```python
from build123d import *

# Parameters (mm, degrees)
F0_W        = 19.1873764305
F0_H        = 101.6
F1_DEPTH    = 76.2
F3_DEPTH    = 67.31
F4_T1_DEPTH = 697.6501262753
F5_R        = 5.07999
F6_R        = 5.08


# Not quite as in the source:
# - a fillet or chamfer that OpenCascade refuses, or shapes differently, is made with other operations: its cross-section is extruded or revolved along the edge and cut away or added
# - a fillet or chamfer is up to 0.001 mm smaller than in the source, because OpenCascade refuses the exact size


with BuildPart() as f1:
    # F0 (on Right) → F1 (new body, symmetric)
    with BuildSketch(Plane.YZ):
        with BuildLine():
            Line((-28.6442058678, -4.364277937), (-36.9899753063, 5.2085028753))
            Line((-36.9899753063, 5.2085028753), (-36.9899753063, -13.8414971247))
            Line((-36.9899753063, -13.8414971247), (39.2100246937, -13.8414971247))
            Line((39.2100246937, -13.8414971247), (39.2100246937, 87.7585028753))
            ThreePointArc((39.2100246937, 87.7585028753), (20.4155377225, 30.5509785676), (-28.6442058678, -4.364277937))
        make_face()
        Polygon((-36.9899753063, -13.8414971247), (-36.9899753063, 5.2085028753), (-36.9899753063, 5.6934356689), (-42.0699753063, 5.6934356689), (-42.0699753063, -13.8414971247), align=None)
        with Locations((48.803712909, 36.9585028753)):
            Rectangle(F0_W, F0_H)
    extrude(amount=F1_DEPTH, both=True)

    # F2 (on Front) → F3 (cut, symmetric)
    with BuildSketch(Plane.XZ):
        with BuildLine():
            ThreePointArc((50.7993000876, -14.1734545694), (0.1539604747, 36.9344649658), (-50.8002333049, -13.8655350342))
            Line((-50.8002333049, -13.8655350342), (50.7993000876, -14.1734545694))
        make_face()
    extrude(amount=F3_DEPTH, both=True, mode=Mode.SUBTRACT)

    # F4: fillet of radius 319.4825375631 on 1 edges, made by hand

    # F4_s2 → F4_t1 (cut)
    with BuildSketch(Plane.YZ.offset(-348.8250631377)):
        with BuildLine():
            ThreePointArc((39.2100246937, 87.7585028753), (53.5639950587, 34.0710629609), (58.3974011242, -21.2915223798))
            Line((58.3974011242, -21.2915223798), (64.7870518755, -21.2915223798))
            Line((64.7870518755, -21.2915223798), (64.7870518755, 87.7585028753))
            Line((64.7870518755, 87.7585028753), (58.3974011242, 94.1481536266))
            ThreePointArc((58.3974011242, 94.1481536266), (48.803712909, 94.1481536266), (45.2159279163, 89.9395033804))
            Line((45.2159279163, 89.9395033804), (39.2100246937, 87.7585028753))
        make_face()
    extrude(amount=F4_T1_DEPTH, mode=Mode.SUBTRACT)

    # F5 (radius 5.08 in the source; OpenCascade refuses exactly that, so slightly less here)
    f5_edges = [f1.edges().sort_by_distance(p)[0] for p in [
        (-61.542005, -42.069975, 5.693436),
        (61.542005, -42.069975, 5.693436),
    ]]
    fillet(f5_edges, radius=F5_R)

    # F6
    f6_edges = [f1.edges().sort_by_distance(p)[0] for p in [
        (0, 39.210025, 87.758503),
    ]]
    fillet(f6_edges, radius=F6_R)


solid = f1.part
```
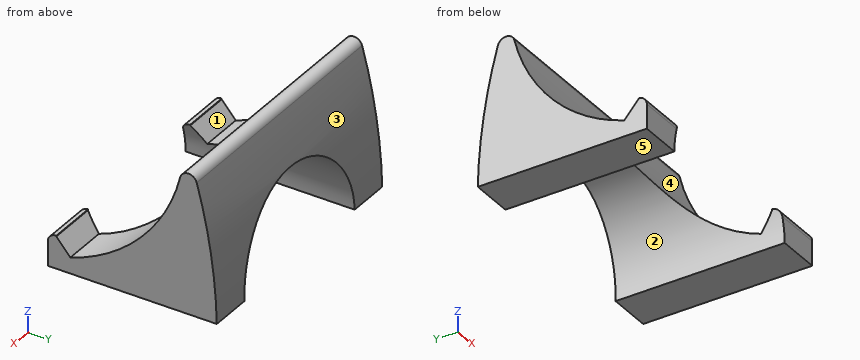
Build history of the part. All positions in model axes, mm. Face numbers are marked on the shaded views. A direction names the side the tool comes from. Round coordinates to 2 decimals unless told otherwise and drop trailing zeros. Write each loop counter-clockwise with the first axis right and the second up, starting at its lowest first coordinate (ties: lowest second). Pieces come first, ordered by that corner, then holes.
1) Band-saw the part on A-A, the plane z = 31. List the corners of the cut face in (x, y).
2) Mould opens along Y. For the marked faces 3, 4 and 5 say: +Y half, -Y half, draft (parallel to the pull), parting line (faces both ways), or undercut.
3) Drill centre lines: probe 1 along X at (y, z) = (24, 22); probe 2 along Y at (x, z) = (-40.5, 47); probe 3 along Y at (x, z) = (68.5, 20.5). Where is each one in solid material? Low to high.
4) Band-saw the part on D-D, the plane z = 49. List the corners of the cut face in (x, y), and give its area (3 significant figures).
5) Band-saw the part on B-B, the plane y = 48. List the corners of the cut face in (x, z).
6) Band-saw the part on C-C, the plane z = 12.5. List the corners of the cut face in (x, y), and give its area (3 significant figures).
7) Pin check, flat tips, straight feed: pin 1 (0.5 mm diameter, centred on x = -63, z = 5.5, fed in from +Y); pin 2 (2 mm diameter, centred on x = 55, z = 59.5, fed in from -Y); pin 3 (8 mm diameter, centred on x = 49, z = 53, fed in from -Y). Stop position of each tip, or through.
8) 3-axis set-ups, long thin cutter, end or side, ignore diameter. For the marked faces 1 and 2: which of +Z, -Z, +X, -X, +Y, -Y reach the whole face in a straight line?
Ans:
1. outline: (-76.2, 20.74) - (-23.83, 20.74) - (-23.83, 54.09) - (-76.2, 54.09) - close; (23.83, 20.74) - (76.2, 20.74) - (76.2, 54.09) - (23.83, 54.09) - close
2. face 3: +Y half
2. face 4: undercut
2. face 5: draft
3. probe 1: x = -76.2 to -35.98, 35.98 to 76.2
3. probe 2: y = 30.18 to 51.01
3. probe 3: y = 11.89 to 55.65
4. outline: (-76.2, 31.08) - (76.2, 31.08) - (76.2, 50.57) - (-76.2, 50.57) - close
4. area: 2,970 mm2
5. outline: (-76.2, -13.84) - (-50.8, -13.84) arc R50.8 cw to (50.8, -13.84) - (76.2, -13.84) - (76.2, 59.55) - (-76.2, 59.55) - close
6. outline: (-76.2, 3.09) - (-43.42, 3.09) - (-43.42, 56.61) - (-76.2, 56.61) - close; (43.42, 3.09) - (76.2, 3.09) - (76.2, 56.61) - (43.42, 56.61) - close
6. area: 3,510 mm2
7. pin 1: stops at y = 57.29
7. pin 2: stops at y = 34.67
7. pin 3: stops at y = 31.08
8. face 1: +Z, +X, -X
8. face 2: -Z, +Y, -Y
